from build123d import *

# Parameters (mm, degrees)
BOX001_W         = 70
BOX001_H         = 10.4
BOX001_DEPTH     = 5.4
ARRAY001_Y_COUNT = 3
ARRAY001_Y_PITCH = 20
ARRAY002_COUNT   = 3
PAD_DEPTH        = 10
SKETCH001_R      = 20.594011
POCKET_DEPTH     = 10.001
FILLET003_R      = 4.9
FILLET004_R      = 4.9


with BuildPart() as array002:
    # Box001 → Box001 (new body)
    with BuildSketch(Plane(origin=(-93.094011, 19.8, 2.3), x_dir=(1, 0, 0), z_dir=(0, 0, 1))):
        with Locations((35, 5.2)):
            Rectangle(BOX001_W, BOX001_H)
    extrude(amount=BOX001_DEPTH)

    # Array001 Y: Array002 ×3


with BuildPart() as array002_1:
    add(array002.part)
    with Locations(*[(0, -i * ARRAY001_Y_PITCH, 0) for i in range(1, ARRAY001_Y_COUNT)]):
        add(array002.part)

    # Array002: Array002 ×3 about axis
    array002_axis = Axis((0, 0, 0), (0, 0, 1))


with BuildPart() as array002_2:
    add(array002_1.part)
    for i in range(1, ARRAY002_COUNT):
        add(array002_1.part.rotate(array002_axis, i * 360 / ARRAY002_COUNT))


with BuildPart() as innerjoinerbase:
    # Sketch (on XY_Plane of Origin) → Pad (new body)
    with BuildSketch(Plane.XY):
        Polygon((-23.094011, 40), (11.905989, 100.621778), (81.188022, 60.621778), (46.188022, 0), (81.188022, -60.621778), (11.905989, -100.621778), (-23.094011, -40), (-93.094011, -40), (-93.094011, 40), align=None)
    extrude(amount=PAD_DEPTH)

    # Sketch001 (on Face11 of Pad) → Pocket (cut, through all)
    with BuildSketch(Plane.XY.offset(10)):
        Circle(SKETCH001_R)
    extrude(amount=-POCKET_DEPTH, mode=Mode.SUBTRACT)

    # Fillet003
    fillet003_edges = [innerjoinerbase.edges().sort_by_distance(p)[0] for p in [
        (-5.594011, -70.310889, 0),
        (-58.094011, -40, 0),
        (-58.094011, -40, 10),
        (-5.594011, -70.310889, 10),
        (-58.094011, 40, 0),
        (-5.594011, 70.310889, 0),
        (-5.594011, 70.310889, 10),
        (-58.094011, 40, 10),
        (63.688022, 30.310889, 10),
        (63.688022, -30.310889, 10),
        (63.688022, -30.310889, 0),
        (63.688022, 30.310889, 0),
        (-23.094011, -40, 5),
        (46.188022, 0, 5),
        (-23.094011, 40, 5),
    ]]
    fillet(fillet003_edges, radius=FILLET003_R)

    # Fillet004
    fillet004_edges = [innerjoinerbase.edges().sort_by_distance(p)[0] for p in [
        (-20.594011, 0, 0),
        (-20.594011, 0, 10),
    ]]
    fillet(fillet004_edges, radius=FILLET004_R)

    # Cut: cut Array002
    add(array002_2.part, mode=Mode.SUBTRACT)


solid = innerjoinerbase.part
Model file for the job. Use its own axes, mm. A direction names the side the tool comes from. Give positions to 0.01 mm unless a question says otherwise; leave off trailing zeros. Order: outer loops, then holes, each group sorted by start corner. A loop starts at its lowest first (then second) coordinate and runs counter-clockwise, first axis right, second up. Notation, with made-up numbers: (71.25, -28) - (110.25, -28) arc R24 cw to (110.25, -11) - close; hole circle Ø5 at (68.5, 82.5). An arc over 180 degrees is marked (long way). Return JSON: item names as keys, results as strings.
1) Pull direction Z, two halves, no side cores. Call faces 4 (the flat face through (12, 23, 0)), 5 (the flat face through (-10.041, -32.464, 4.962)), 6 (the cylindrical face through (-59.98, -38.53, 8.6)): pulls with the +Z half, pulls with the -Z half, needs draft (parallel to the pull), parting line crosses it, or undercut.
Geometry says:
{"face 4": "pulls with the -Z half", "face 5": "undercut", "face 6": "pulls with the +Z half"}
2) 3-axis set-ups, long thin cutter, end or side, ignore diameter. For faces 1 (the flat face through (-59, 5, 7.7)), 2 (the flat face through (15.81, 17.54, 4.96)), 3 (the cylindrical face through (-59.04, 38.6, 1.47)): which of +Z, -Z, +X, -X, +Y, -Y reach the whole face in a straight line?
Geometry says:
{"face 1": "-X", "face 2": "none", "face 3": "-Z, -X, +Y"}
3) Cut at A-A, the plane x = -61. Give the cut face in (y, z).
Geometry says:
{"outline": "(-40, 4.9) arc R4.9 ccw to (-35.1, 0) - (35.1, 0) arc R4.9 ccw to (40, 4.9) - (40, 5.1) arc R4.9 ccw to (35.1, 10) - (-35.1, 10) arc R4.9 ccw to (-40, 5.1) - close; hole (-20.2, 2.3) - (-9.8, 2.3) - (-9.8, 7.7) - (-20.2, 7.7) - close; hole (-0.2, 2.3) - (10.2, 2.3) - (10.2, 7.7) - (-0.2, 7.7) - close; hole (19.8, 2.3) - (30.2, 2.3) - (30.2, 7.7) - (19.8, 7.7) - close"}
4) Cut at B-B, the plane x = 0. Count the separate pieces of the cut face and the enclosed holes in it, plus the area to 3 significant figures.
Geometry says:
{"separate pieces": "2", "enclosed holes": "2", "area": "940 mm²"}
5) Flat gauge pins, fed straight in: P1, Ø1.6, axis at x = -41, z = 4, coming from the +Y side; P2, Ø3, axis at x = 50.5, z = 7, coming from the +Y side; P3, Ø10, axis at x = -12.5, y = -69, coming from the +Z side; P4, Ø6, axis at y = 4.5, z = 5.5, coming from the -X side. Where does each tip first touch, or does it go through?
Geometry says:
{"P1": "y = 40", "P2": "y = 79.11", "P3": "through", "P4": "x = -93.09"}
6) Probe line 1 (Y direction, x = -8, z = 7.5); line 2 (Z direction, x = -57.5, y = -17); line 3 (Y direction, x = 25, z = 7.25). List the from-to ranges inside material, lowest first. Write a range as from..to.
Geometry says:
{"line 1": "-64.89..-46.54, -31.29..-19.66, 19.66..64.89", "line 2": "0..2.3, 7.7..10", "line 3": "-82.9..-63.7, -42.9..-23.7, -12.23..22.9, 43.7..62.9, 83.7..93.06"}
